from build123d import *

# Parameters (mm, degrees)
SKETCH1_W           = 60
SKETCH1_H           = 80
BOSS_EXTRUDE1_DEPTH = 6
SKETCH2_R           = 2.55
CUT_EXTRUDE1_DEPTH  = 51.358713248
SKETCH3_W           = 10
SKETCH3_H           = 6
BOSS_EXTRUDE2_DEPTH = 20


with BuildPart() as part:
    # Sketch1 → Boss-Extrude1 (new body)
    with BuildSketch(Plane(origin=(0, 0, 0), x_dir=(1, 0, 0), z_dir=(0, 1, 0))):
        Rectangle(SKETCH1_W, SKETCH1_H)
    extrude(amount=BOSS_EXTRUDE1_DEPTH)

    # Sketch2 → Cut-Extrude1 (cut, through all)
    with BuildSketch(Plane(origin=(0, 6, 0), x_dir=(1, 0, 0), z_dir=(0, 1, 0))):
        with Locations(Location((25, -9, 0), (0, 0, 270))):
            Circle(SKETCH2_R)
        with Locations(Location((-25, -9, 0), (0, 0, 270))):
            Circle(SKETCH2_R)
        with Locations(Location((0, -29, 0), (0, 0, 270))):
            Circle(SKETCH2_R)
        Polygon((-38.891606185, 9), (-20, 9), (-20, 19), (20, 19), (20, 9), (37.945141675, 9), (37.945141675, 57.336722716), (-38.891606185, 57.336722716), align=None)
    extrude(amount=-CUT_EXTRUDE1_DEPTH, mode=Mode.SUBTRACT)

    # Sketch3 → Boss-Extrude2 (add)
    with BuildSketch(Plane(origin=(0, 6, 0), x_dir=(1, 0, 0), z_dir=(0, 1, 0))):
        with Locations((25, 6)):
            Rectangle(SKETCH3_W, SKETCH3_H)
        with Locations((-25, 6)):
            Rectangle(SKETCH3_W, SKETCH3_H)
    extrude(amount=BOSS_EXTRUDE2_DEPTH)


solid = part.part
Here's how the part is built. I have some questions about the finished solid (model axes, mm). A direction names the side the tool comes from. Coordinates: 2 decimals unless noted, no trailing zeros. Loops run counter-clockwise (first coordinate to the right, second up) from the corner with the lowest first, then second, coordinate; pieces in that order, holes last.
1. Imagine slicing it at C-C, the plane y = 3. Please give me the cut outline in (x, z), and give its area (3 significant figures).
2. Imagine slicing it at A-A, the plane z = 29. Please give me the cut outline in (x, y).
3. Imagine slicing it at D-D, the plane z = 9. Please give me the cut outline in (x, y).
4. For P1, Ø8, axis at x = 16.5, y = 19.5, coming from the -Z side; P2, Ø3, axis at x = 22.5, y = 17.5, coming from the +Z side; P3, Ø1.8, axis at y = 4, z = -16.5, coming from the +X side; P4, Ø6.5, axis at x = 0, z = 29, coming from the -Y side, each with a flat end and sliding along its axis, tell me the tip position at first contact or that it passes through.
5. Imagine slicing it at B-B, the plane x = 0. Please give me the cut outline in (y, z), and give its area (3 significant figures).
6. If we mould it in two halves opening along X, with no side actions, what happens to faces 1 (the cylindrical face through (-24.23, 3.04, 11.43)), 2 (the flat face through (25, 16, -3)), 3 (the flat face through (30, 4, 8)), 4 (the cylindrical face through (0.112, 3.042, 26.452))? For each: pulls with the +X half, pulls with the -X half, needs draft (parallel to the pull), parting line crosses it, or undercut.
7. I need wall thicknesses on L1, parallel to X at y = 3.1, z = 9; L2, parallel to X at y = 10, z = -4; L3, parallel to X at y = 4.45, z = 29. Which ranges of each line are inside material? Lowest first, please.
8. For faces 5 (the flat face through (20, 16, -6)), 6 (the flat face through (-20, 3, -14)), 7 (the flat face through (0, 3, -19)), 8 (the flat face through (25, 13, -9)), 9 (the flat face through (-25, 16, -3)), which set-ups out of +Z, -Z, +X, -X, +Y, -Y let a thin tool reach every point of the face, with its end or its side?
Taken from the geometry:
1. outline: (-30, -9) - (-20, -9) - (-20, -19) - (20, -19) - (20, -9) - (30, -9) - (30, 40) - (-30, 40) - close; hole circle Ø5.1 at (-25, 9); hole circle Ø5.1 at (0, 29); hole circle Ø5.1 at (25, 9)
1. area: 3,280 mm2
2. outline: (-30, 0) - (-2.55, 0) - (-2.55, 6) - (-30, 6) - close; (2.55, 0) - (30, 0) - (30, 6) - (2.55, 6) - close
3. outline: (-30, 0) - (-27.55, 0) - (-27.55, 6) - (-30, 6) - close; (-22.45, 0) - (22.45, 0) - (22.45, 6) - (-22.45, 6) - close; (27.55, 0) - (30, 0) - (30, 6) - (27.55, 6) - close
4. P1: stops at z = -9
4. P2: stops at z = -3
4. P3: stops at x = 20
4. P4: stops at y = 0
5. outline: (0, -19) - (6, -19) - (6, 26.45) - (0, 26.45) - close; (0, 31.55) - (6, 31.55) - (6, 40) - (0, 40) - close
5. area: 323 mm2
6. face 1: undercut
6. face 2: needs draft
6. face 3: pulls with the +X half
6. face 4: undercut
7. L1: x = -30 to -27.55, -22.45 to 22.45, 27.55 to 30
7. L2: x = -30 to -20, 20 to 30
7. L3: x = -30 to -2.55, 2.55 to 30
8. face 5: +Z, -Z, +Y
8. face 6: -Z, -X, +Y, -Y
8. face 7: -Z, +X, -X, +Y, -Y
8. face 8: -Z, +X, +Y, -Y
8. face 9: +Z, +X, -X, +Y
